For this review, use the dimensioned drawing (mm, ordinates from the lowest corner) and the shaded views. Give positions to 0.01 mm unless a question says otherwise; leave off trailing zeros. Loops run counter-clockwise (first coordinate to the right, second up) from the corner with the lowest first, then second, coordinate; pieces in that order, holes last. Notation, with made-up numbers: M 22,-14.75 L 32,-14.75 A28 ccw 32,4.25 Z; hole C 35,64 d9. An arc over 180 degrees is marked long. Use a Markdown table: item, result. Add a question column.
(1) Add section B-B, the plane z = 25. Give the boundary of the cut face in (x, y).
(2) For probe 1 along X at (y, z) = (7.5, 26); probe 2 along X at (y, z) = (17.5, 43); probe 3 along Y at (x, z) = (27, 23), list the stretches that pass through material, from the lowest coordinate up.
(3) Add section A-A, the plane y = 15. Give the boundary of the cut face in (x, z).
(4) Insertion check: pin 1 Ø10 at (y, z) = (5, 66) entering from -X; pin 2 Ø6 at (x, y) = (1.5, 15) entering from +Z; pin 3 Ø1.4 at (x, z) = (4, 7.5) entering from +Y. Each pin has a flat end and moves straight along its axis. Give the tip position at first contact, or say it passes through.
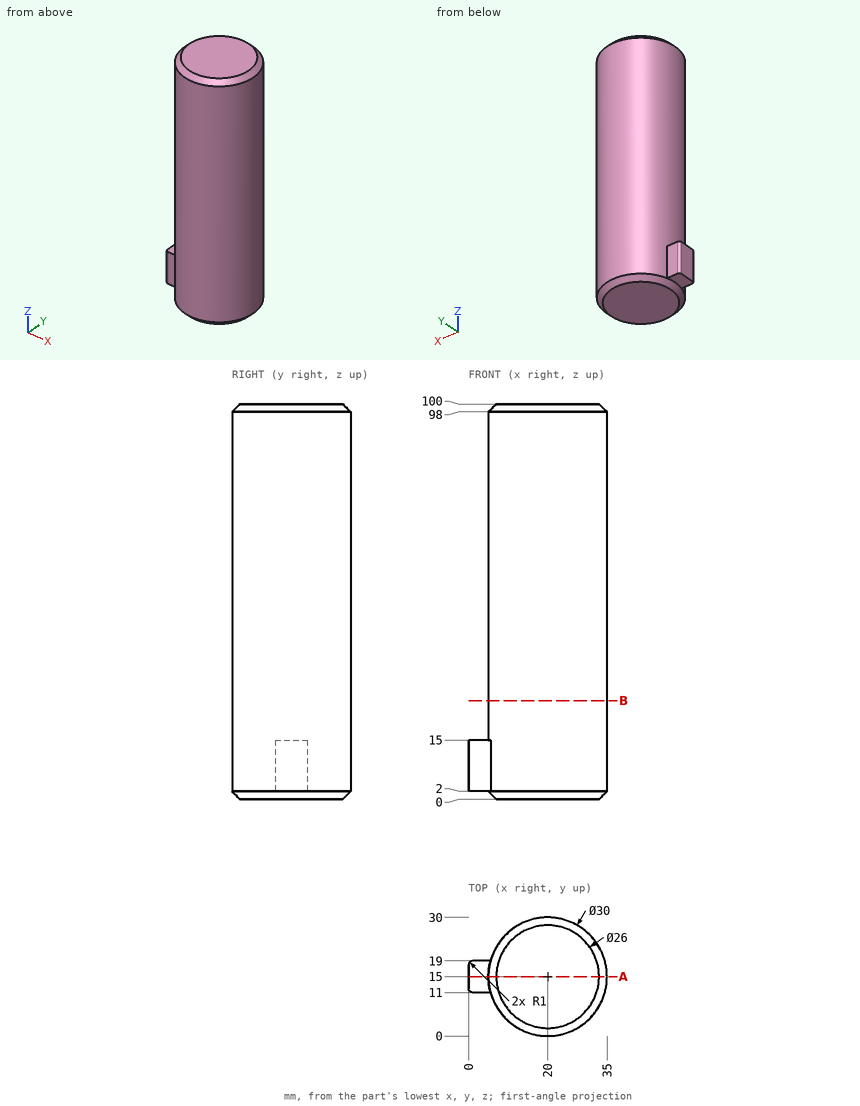
Established:
| question | item | result |
|---|---|---|
| 1 | outline | C 20,15 d30 |
| 2 | probe 1 | 7.01 to 32.99 |
| 2 | probe 2 | 5.21 to 34.79 |
| 2 | probe 3 | 1.73 to 28.27 |
| 3 | outline | M 0,2 L 5,2 L 7,0 L 33,0 L 35,2 L 35,98 L 33,100 L 7,100 L 5,98 L 5,15 L 0,15 Z |
| 4 | pin 1 | x = 5.86 |
| 4 | pin 2 | z = 15 |
| 4 | pin 3 | y = 19 |
